from build123d import *

# Parameters (mm, degrees)
F1_DEPTH = 25
F0_W     = 3.1244163401
F0_H     = 10
F0_W_2   = 3
F2_DEPTH = 25
F3_W     = 3.4
F3_H     = 4
F3_W_2   = 5
F3_H_2   = 7.5
F4_DEPTH = 25


# Not quite as in the source:
# - a feature names something its author has since deleted; it is built from what else it names


with BuildPart() as f1:
    # F0 (on Top) → F1 (new body)
    with BuildSketch(Plane.XY):
        with BuildLine():
            Line((4.5, 0), (0, 0))
            Line((0, 0), (0, 15))
            Line((0, 15), (1, 15))
            Line((1, 15), (0, 16))
            Line((0, 16), (-3.1244163401, 16))
            Line((-3.1244163401, 16), (-3.1244163401, 15))
            Line((-3.1244163401, 15), (-3.1244163401, 0))
            Line((-3.1244163401, 0), (-3.1244163401, -5))
            ThreePointArc((-3.1244163401, -5), (-2.8315231213, -5.7071067812), (-2.1244163401, -6))
            Line((-2.1244163401, -6), (4.5, -6))
            Line((4.5, -6), (6.5, -6))
            ThreePointArc((6.5, -6), (7.2071067812, -5.7071067812), (7.5, -5))
            Line((7.5, -5), (7.5, 15))
            Line((7.5, 15), (7.5, 16))
            Line((7.5, 16), (4.5, 16))
            Line((4.5, 16), (3.5, 15))
            Line((3.5, 15), (4.5, 15))
            Line((4.5, 15), (4.5, 0))
        make_face()
    extrude(amount=F1_DEPTH)

    # F0 (on Top) → F2 (join)
    with BuildSketch(Plane.XY):
        with BuildLine():
            Line((4.5, 0), (0, 0))
            Line((0, 0), (0, 15))
            Line((0, 15), (1, 15))
            Line((1, 15), (0, 16))
            Line((0, 16), (-3.1244163401, 16))
            Line((-3.1244163401, 16), (-3.1244163401, 15))
            Line((-3.1244163401, 15), (-3.1244163401, 0))
            Line((-3.1244163401, 0), (-3.1244163401, -5))
            ThreePointArc((-3.1244163401, -5), (-2.8315231213, -5.7071067812), (-2.1244163401, -6))
            Line((-2.1244163401, -6), (4.5, -6))
            Line((4.5, -6), (6.5, -6))
            ThreePointArc((6.5, -6), (7.2071067812, -5.7071067812), (7.5, -5))
            Line((7.5, -5), (7.5, 15))
            Line((7.5, 15), (7.5, 16))
            Line((7.5, 16), (4.5, 16))
            Line((4.5, 16), (3.5, 15))
            Line((3.5, 15), (4.5, 15))
            Line((4.5, 15), (4.5, 0))
        make_face()
        with Locations((-1.5622081701, 21)):
            Rectangle(F0_W, F0_H)
        with Locations((6, 21)):
            Rectangle(F0_W_2, F0_H)
    extrude(amount=F2_DEPTH)

    # F3 (on face) → F4 (cut)
    with BuildSketch(Plane.YZ.offset(7.5)):
        with Locations((22.7, 12.5)):
            Rectangle(F3_W, F3_H)
        with Locations((23.5, 21.25)):
            Rectangle(F3_W_2, F3_H_2)
        with Locations((22.7, 3.75)):
            Rectangle(F3_W, F3_H_2)
    extrude(amount=-F4_DEPTH, mode=Mode.SUBTRACT)


solid = f1.part
The listing builds one solid part. Answer for the finished solid, in the listing's coordinates (mm). A direction names the side the tool comes from. Round coordinates to 2 decimals unless told otherwise and drop trailing zeros. Order: outer loops, then holes, each group sorted by start corner. A loop starts at its lowest first (then second) coordinate and runs counter-clockwise, first axis right, second up. Notation, with made-up numbers: (-18.5, -13) - (11.5, -13) arc R31 cw to (11.5, 22) - close; hole circle Ø8 at (21.25, 54.25). An arc over 180 degrees is marked (long way). Write item = value, one per line. Start each with the question number.
1) Section D-D, the plane z = 22.25 is taken. Write down the section's boundary in (x, y).
2) Given pin 1 (1.6 mm diameter, centred on x = -1.5, y = 23.5, fed in from -Z); pin 2 (1.5 mm diameter, centred on x = 5.5, z = 19.5, fed in from +Y); pin 3 (1.3 mm diameter, centred on x = 3, z = 16.5, fed in from +Y), each flat-ended and moving along its own axis, determine where each tip first touches the part or whether it passes through.
3) Straight lines are drawn through the part: L1, parallel to X at y = 13.5, z = 17.25; L2, parallel to Y at x = 4.75, z = 10.75; L3, parallel to Y at x = 4.75, z = 20.5. For each, find the intervals that lie inside material, in ascending order.
4) For a pull along Z with two mould halves and no side action, classify faces 1 (the flat face through (6, 21, 4)), 2 (the flat face through (6, 21, 12)), 3 (the flat face through (6, 25, 0)) as released by +Z, released by -Z, zero draft, split by the parting line, or undercut.
5) Section A-A, the plane y = 18 is taken. Write down the section's boundary in (x, z).
6) Section C-C, the plane x = 0.5 is taken. Write down the section's boundary in (y, z), plus the area to 4 significant figures.
7) For faces 4 (the flat face through (6, 23, 10.5)), 5 (the flat face through (-2, 23, 7.5)), 6 (the flat face through (-2, 21, 21)), 7 (the flat face through (4, 15.5, 12.3)), 8 (the flat face through (0, 7, 12)), determine the directions among +Z, -Z, +X, -X, +Y, -Y from which every point of the face is accessible in a straight line to the end or side of a thin tool.
8) Section B-B, the plane z = 7 is taken. Write down the section's boundary in (x, y), plus the area to 3 significant figures.
Results list:
q1.outline = (-3.12, -5) arc R1 ccw to (-2.12, -6) - (6.5, -6) arc R1 ccw to (7.5, -5) - (7.5, 21) - (4.5, 21) - (4.5, 16) - (3.5, 15) - (4.5, 15) - (4.5, 0) - (0, 0) - (0, 15) - (1, 15) - (0, 16) - (0, 21) - (-3.12, 21) - close
q2.pin_1 = 7.5
q2.pin_2 = 21
q2.pin_3 = 15.15
q3.L1 = -3.12 to 0, 4.5 to 7.5
q3.L2 = -6 to 21, 24.4 to 26
q3.L3 = -6 to 21
q4.face_1 = zero draft
q4.face_2 = undercut
q4.face_3 = released by -Z
q5.outline = (-3.12, 0) - (0, 0) - (0, 25) - (-3.12, 25) - close; (4.5, 0) - (7.5, 0) - (7.5, 25) - (4.5, 25) - close
q6.outline = (-6, 0) - (0, 0) - (0, 25) - (-6, 25) - close; (15, 0) - (15.5, 0) - (15.5, 25) - (15, 25) - close
q6.area = 162.5 mm^2
q7.face_4 = +X, -X
q7.face_5 = -Z, +X, -X
q7.face_6 = +Z, +X, -X, +Y
q7.face_7 = +Z, -Z, +Y
q7.face_8 = +Z, -Z
q8.outline = (-3.12, -5) arc R1 ccw to (-2.12, -6) - (6.5, -6) arc R1 ccw to (7.5, -5) - (7.5, 21) - (4.5, 21) - (4.5, 16) - (3.5, 15) - (4.5, 15) - (4.5, 0) - (0, 0) - (0, 15) - (1, 15) - (0, 16) - (0, 21) - (-3.12, 21) - close; (-3.12, 24.4) - (0, 24.4) - (0, 26) - (-3.12, 26) - close; (4.5, 24.4) - (7.5, 24.4) - (7.5, 26) - (4.5, 26) - close
q8.area = 203 mm^2
